```python
from build123d import *

# Parameters (mm, degrees)
SKETCH1_W           = 63.5
SKETCH1_H           = 31.75
SKETCH1_R           = 4.7625
BOSS_EXTRUDE1_DEPTH = 19.05
SKETCH1_3_R         = 4.7625
SKETCH1_3_R_2       = 2.5527
BOSS_EXTRUDE2_DEPTH = 14.224


with BuildPart() as part:
    # Sketch1 → Boss-Extrude1 (new body)
    with BuildSketch(Plane.XY):
        with Locations((4.146938776, -4.146938776)):
            Rectangle(SKETCH1_W, SKETCH1_H)
        with Locations(Location((29.546938776, -13.671938776, 0), (0, 0, 180))):
            Circle(SKETCH1_R, mode=Mode.SUBTRACT)
        with Locations(Location((-21.253061224, -13.671938776, 0), (0, 0, 180))):
            Circle(SKETCH1_R, mode=Mode.SUBTRACT)
    extrude(amount=BOSS_EXTRUDE1_DEPTH)

    # Sketch1_3 → Boss-Extrude2 (add)
    # profile 1 of 2: a face of its own
    with BuildSketch(Plane.XY):
        with Locations(Location((-21.253061224, -13.671938776, 0), (0, 0, 180))):
            Circle(SKETCH1_3_R)
        with Locations((-21.253061224, -13.671938776)):
            Circle(SKETCH1_3_R_2, mode=Mode.SUBTRACT)
    # profile 2 of 2: a face of its own
    with BuildSketch(Plane.XY):
        with Locations(Location((29.546938776, -13.671938776, 0), (0, 0, 180))):
            Circle(SKETCH1_3_R)
        with Locations((29.546938776, -13.671938776)):
            Circle(SKETCH1_3_R_2, mode=Mode.SUBTRACT)
    extrude(amount=BOSS_EXTRUDE2_DEPTH)


solid = part.part
```
Model file for the job. Use its own axes, mm. A direction names the side the tool comes from. Round coordinates to 2 decimals unless told otherwise and drop trailing zeros. Loops run counter-clockwise (first coordinate to the right, second up) from the corner with the lowest first, then second, coordinate; pieces in that order, holes last. Notation, with made-up numbers: M 60,-25.5 L 77,-25.5 A32 ccw 77,4.5 Z; hole C 33,49.25 d8. An arc over 180 degrees is marked long. Put each result on its own line as item: value. Start each with the question number.
Item 1: Mould opens along X. For faces 1 (the face through (35.897, -4, 9)), 2 (the face through (-21.806, -16.164, 7.012)), 3 (the face through (4, -20.022, 9)) say: released by +X, released by -X, zero draft, split by the parting line, or undercut.
Item 2: Cut at D-D (y = -17.5). List the corners of the cut face in (x, z), then the cut area to 3 significant figures.
Item 3: Cut at A-A (x = -23). List the corners of the cut face in (y, z), then the cut area to 3 significant figures.
Item 4: 3-axis set-ups, long thin cutter, end or side, ignore diameter. For faces 4 (the face through (5, -4, 0)), 5 (the face through (-23.451, -9.447, 16.603)): which of +Z, -Z, +X, -X, +Y, -Y reach the whole face in a straight line?
Item 5: Cut at B-B (y = -12). List the corners of the cut face in (x, z).
Item 6: Drop flat-ended pins along their axis: P1, Ø3, axis at x = 29.55, y = -13.67, coming from the +Z side; P2, Ø6, axis at x = -21.25, y = -13.67, coming from the +Z side. Give the stop position or say it passes through.
Item 7: Cut at C-C (z = 11.5). List the corners of the cut face in (x, y).
Item 8: Drill centre lines: line 1 along X through (y, z) = (-14, 3.75); line 2 along X through (y, z) = (-16, 13); line 3 along Y through (x, z) = (-22.5, 16.5). Where is each one in solid material? Low to high.
Answer block:
1. face 1: released by +X
1. face 2: undercut
1. face 3: zero draft
2. outline: M -27.6,0 L 35.9,0 L 35.9,19.05 L 32.38,19.05 L 32.38,14.22 L 26.71,14.22 L 26.71,19.05 L -18.42,19.05 L -18.42,14.22 L -24.09,14.22 L -24.09,19.05 L -27.6,19.05 Z
2. area: 1,150 mm2
3. outline: M -20.02,0 L -15.53,0 L -15.53,14.22 L -18.1,14.22 L -18.1,19.05 L -20.02,19.05 Z; M -11.81,0 L 11.73,0 L 11.73,19.05 L -9.24,19.05 L -9.24,14.22 L -11.81,14.22 Z
3. area: 509 mm2
4. face 4: -Z, +X, -X, +Y, -Y
4. face 5: +Z
5. outline: M -27.6,0 L -23.18,0 L -23.18,14.22 L -25.71,14.22 L -25.71,19.05 L -27.6,19.05 Z; M -19.32,0 L 27.62,0 L 27.62,14.22 L 25.09,14.22 L 25.09,19.05 L -16.79,19.05 L -16.79,14.22 L -19.32,14.22 Z; M 31.48,0 L 35.9,0 L 35.9,19.05 L 34.01,19.05 L 34.01,14.22 L 31.48,14.22 Z
6. P1: through
6. P2: z = 14.22
7. outline: M -27.6,-20.02 L 35.9,-20.02 L 35.9,11.73 L -27.6,11.73 Z; hole C -21.25,-13.67 d5.11; hole C 29.55,-13.67 d5.11
8. line 1: -27.6 to -23.78, -18.72 to 27.02, 32.08 to 35.9
8. line 2: -27.6 to -22.3, -20.21 to 28.5, 30.59 to 35.9
8. line 3: -20.02 to -18.27, -9.08 to 11.73
